For this review, use the dimensioned drawing (mm, ordinates from the lowest corner) and the shaded views. Coordinates: 2 decimals unless noted, no trailing zeros. Write each loop counter-clockwise with the first axis right and the second up, starting at its lowest first coordinate (ties: lowest second). Pieces come first, ordered by that corner, then holes. Notation, with made-up numbers: M 3.5,55 L 7.5,55 A20 ccw 7.5,84 Z; hole C -25,42 d5. An arc over 180 degrees is marked long. Return JSON: item names as keys, results as strings. Group by question number.
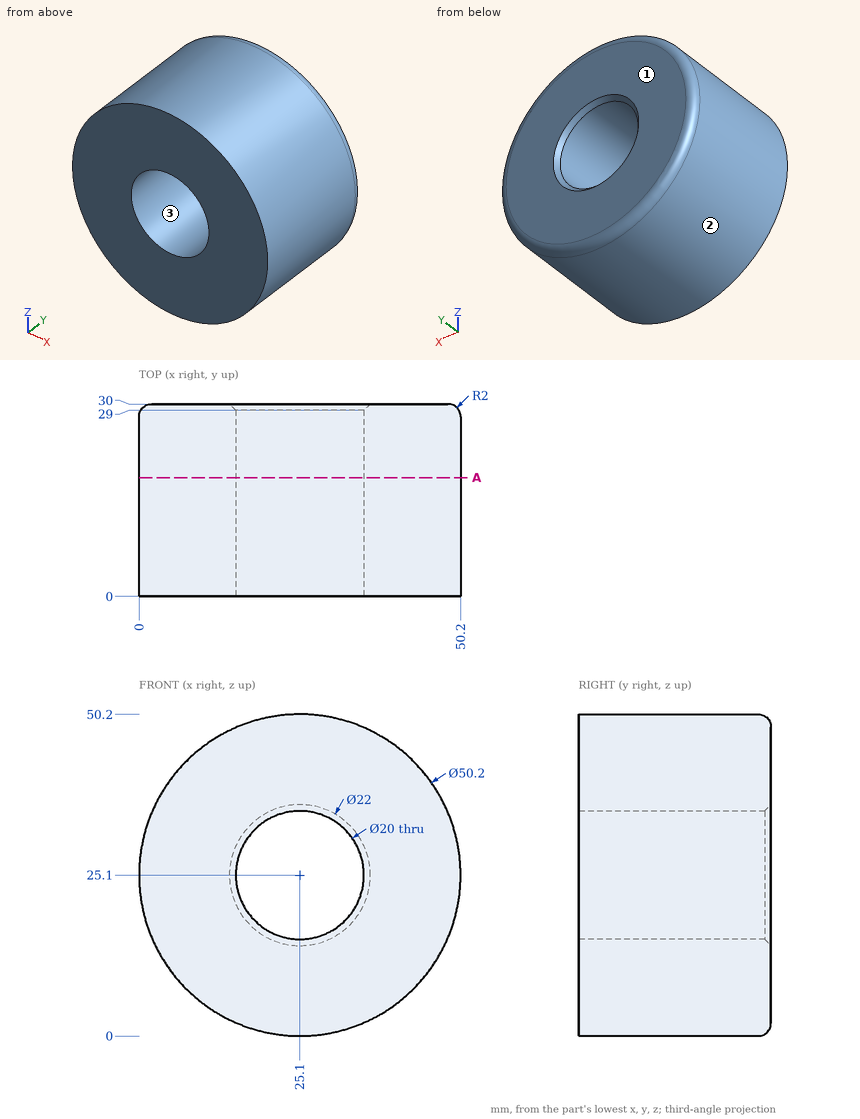
Item 1: The part is to be moulded in two halves that separate along X. For the marked faces 1, 2 and 3, say which applies: pulls with the +X half, pulls with the -X half, needs draft (parallel to the pull), parting line crosses it, or undercut.
Item 2: Add section A-A (y = 18.5). Write out the cut boundary in (x, z).
Item 3: For pin 1 (8 mm diameter, centred on y = 14.5, z = 38.5, fed in from -X); pin 2 (8 mm diameter, centred on x = 29, y = 19.5, fed in from +Z); pin 3 (1 mm diameter, centred on x = 42, y = 14.5, fed in from -Z), all flat-tipped, find the tip position at first contact; note any pin that passes through.
Item 4: For line 1 (Z direction, x = 25.1, y = 17); line 2 (X direction, y = 10.75, z = 22.5); line 3 (X direction, y = 27.5, z = 16), list the stretches that pass through material, from the lowest coordinate up.
Geometry check:
{
 "1": {"face 1": "needs draft", "face 2": "parting line crosses it", "face 3": "undercut"},
 "2": {"outline": "C 25.1,25.1 d50.2; hole C 25.1,25.1 d20"},
 "3": {"pin 1": "x = 1.83", "pin 2": "z = 50.2", "pin 3": "z = 6.1"},
 "4": {"line 1": "0 to 15.1, 35.1 to 50.2", "line 2": "0.14 to 15.44, 34.76 to 50.06", "line 3": "1.71 to 20.95, 29.25 to 48.49"}
}
